from build123d import *

# Parameters (mm, degrees)
SKETCH1_R           = 4
BOSS_EXTRUDE1_DEPTH = 6
BOSS_EXTRUDE2_DEPTH = 3
SKETCH3_R           = 2.5
CUT_EXTRUDE1_DEPTH  = 12.169153952


with BuildPart() as part:
    # Sketch1 → Boss-Extrude1 (new body)
    with BuildSketch(Plane(origin=(0, 0, 0), x_dir=(1, 0, 0), z_dir=(0, 1, 0))):
        with Locations(Location((0, 0, 0), (0, 0, 270))):
            Circle(SKETCH1_R)
    extrude(amount=BOSS_EXTRUDE1_DEPTH)

    # Sketch2 → Boss-Extrude2 (add)
    with BuildSketch(Plane(origin=(0, 6, 0), x_dir=(1, 0, 0), z_dir=(0, 1, 0))):
        Polygon((2.5, -4.330127019), (5, 0), (2.5, 4.330127019), (-2.5, 4.330127019), (-5, 0), (-2.5, -4.330127019), align=None)
    extrude(amount=BOSS_EXTRUDE2_DEPTH)

    # Sketch3 → Cut-Extrude1 (cut, through all)
    with BuildSketch(Plane(origin=(0, 9, 0), x_dir=(1, 0, 0), z_dir=(0, 1, 0))):
        with Locations(Location((0, 0, 0), (0, 0, 270))):
            Circle(SKETCH3_R)
    extrude(amount=-CUT_EXTRUDE1_DEPTH, mode=Mode.SUBTRACT)


solid = part.part
Read the model definition and answer for the solid it produces. Units are mm, in the model's axes. Round coordinates to 2 decimals unless told otherwise and drop trailing zeros. Loops run counter-clockwise (first coordinate to the right, second up) from the corner with the lowest first, then second, coordinate; pieces in that order, holes last.
Q1. Section C-C on y = 7 is taken. Write down the section's boundary in (x, z), and give its area (3 significant figures).
Q2. Section D-D on x = -3.75 is taken. Write down the section's boundary in (y, z).
Q3. Section B-B on z = -2 is taken. Write down the section's boundary in (x, y).
Q4. Section A-A on x = 0 is taken. Write down the section's boundary in (y, z).
Q5. Consider probe 1 along X at (y, z) = (3, 0); probe 2 along Z at (x, y) = (1.25, 3.25); probe 3 along Y at (x, z) = (1.5, 3.75). Determine where each line is inside the solid, lowest interval first.
Q6. This flat-tipped pin is pushed along its axis until it touches: pin 1 (4.5 mm diameter, centred on x = 0, z = 0, fed in from -Y). Where does it stop, or does it pass through?
Q7. Determine the mould class of faces 1 (the face through (-2.44, 4.56, -0.54)), 2 (the face through (0, 7, -4.33)), 3 (the face through (4.1, 6, -0.7)), 4 (the face through (-3.905, 2.958, -0.867)) for opening direction Z: released by +Z, released by -Z, zero draft, split by the parting line, or undercut.
Output:
1. outline: (-5, 0) - (-2.5, -4.33) - (2.5, -4.33) - (5, 0) - (2.5, 4.33) - (-2.5, 4.33) - close; hole circle Ø5 at (0, 0)
1. area: 45.3 mm2
2. outline: (0, -1.39) - (6, -1.39) - (6, -2.17) - (9, -2.17) - (9, 2.17) - (6, 2.17) - (6, 1.39) - (0, 1.39) - close
3. outline: (-3.85, 6) - (-3.46, 6) - (-3.46, 0) - (-1.5, 0) - (-1.5, 9) - (-3.85, 9) - close; (1.5, 0) - (3.46, 0) - (3.46, 6) - (3.85, 6) - (3.85, 9) - (1.5, 9) - close
4. outline: (0, -4) - (6, -4) - (6, -4.33) - (9, -4.33) - (9, -2.5) - (0, -2.5) - close; (0, 2.5) - (9, 2.5) - (9, 4.33) - (6, 4.33) - (6, 4) - (0, 4) - close
5. probe 1: x = -4 to -2.5, 2.5 to 4
5. probe 2: z = -3.8 to -2.17, 2.17 to 3.8
5. probe 3: y = 6 to 9
6. pin 1: passes through
7. face 1: undercut
7. face 2: released by -Z
7. face 3: zero draft
7. face 4: split by the parting line
